from build123d import *

# Parameters (mm, degrees)
BOSS_EXTRUDE1_DEPTH     = 2.5
CUT_EXTRUDE1_DEPTH      = 37.962819157
CUT_EXTRUDE1_DEPTH_BACK = 37.962819157
SKETCH2_R               = 1


with BuildPart() as part:
    # Sketch1 → Boss-Extrude1 (new, symmetric)
    with BuildSketch(Plane(origin=(0, 0, 0), x_dir=(1, 0, 0), z_dir=(0, 1, 0))):
        Polygon((13, -6), (13, -8), (18, -8), (18, 8), (-18, 8), (-18, -8), (-13, -8), (-13, -6), (-16, -6), (-16, 6), (16, 6), (16, -6), align=None)
    extrude(amount=BOSS_EXTRUDE1_DEPTH, both=True)

    # Sketch2 → Cut-Extrude1 (cut, two sides: drawn at the far end of the back side and taken through both)
    with BuildSketch(Plane(origin=(18, 0, 0), x_dir=(0, 0, -1), z_dir=(1, 0, 0)).offset(-CUT_EXTRUDE1_DEPTH_BACK)):
        Circle(SKETCH2_R)
    extrude(amount=CUT_EXTRUDE1_DEPTH + CUT_EXTRUDE1_DEPTH_BACK, mode=Mode.SUBTRACT)


solid = part.part
CAD build for the part. Positions are in the model's coordinates, mm. A direction names the side the tool comes from. Give positions to 0.01 mm unless a question says otherwise; leave off trailing zeros. Write each loop counter-clockwise with the first axis right and the second up, starting at its lowest first coordinate (ties: lowest second). Pieces come first, ordered by that corner, then holes. Notation, with made-up numbers: (-3.5, 31.5) -> (15.5, 31.5) arc R12 cw to (15.5, 54.5) -> close; hole circle Ø8 at (-36, 9). An arc over 180 degrees is marked (long way). Return JSON: item names as keys, results as strings.
Item 1: Two-plate mould, pull along Z, no slides. Class faces 4 (the flat face through (-18, 1.15, -0.11)), 5 (the flat face through (15, 0, 8)), 6 (the flat face through (15, 0, 6)): +Z half, -Z half, draft (parallel to the pull), parting line (faces both ways), or undercut.
Answer below:
{"face 4": "draft", "face 5": "+Z half", "face 6": "undercut"}
Item 2: Band-saw the part on C-C (y = 0). List the corners of the cut face in (x, z).
Answer below:
{"outline": "(-18, -8) -> (18, -8) -> (18, -1) -> (16, -1) -> (16, -6) -> (-16, -6) -> (-16, -1) -> (-18, -1) -> close; (-18, 1) -> (-16, 1) -> (-16, 6) -> (-13, 6) -> (-13, 8) -> (-18, 8) -> close; (13, 6) -> (16, 6) -> (16, 1) -> (18, 1) -> (18, 8) -> (13, 8) -> close"}
Item 3: Band-saw the part on D-D (x = 4.5). List the corners of the cut face in (y, z).
Answer below:
{"outline": "(-2.5, -8) -> (2.5, -8) -> (2.5, -6) -> (-2.5, -6) -> close"}
Item 4: Drill centre lines: probe 1 along X at (y, z) = (-0.25, 2); probe 2 along Z at (x, y) = (17.2, 0); probe 3 along Y at (x, z) = (16.7, 0). Where is each one in solid material? Low to high.
Answer below:
{"probe 1": "x = -18 to -16, 16 to 18", "probe 2": "z = -8 to -1, 1 to 8", "probe 3": "y = -2.5 to -1, 1 to 2.5"}
Item 5: Band-saw the part on A-A (z = 0). List the corners of the cut face in (x, y).
Answer below:
{"outline": "(-18, -2.5) -> (-16, -2.5) -> (-16, -1) -> (-18, -1) -> close; (-18, 1) -> (-16, 1) -> (-16, 2.5) -> (-18, 2.5) -> close; (16, -2.5) -> (18, -2.5) -> (18, -1) -> (16, -1) -> close; (16, 1) -> (18, 1) -> (18, 2.5) -> (16, 2.5) -> close"}
Item 6: Band-saw the part on B-B (x = 14). List the corners of the cut face in (y, z), then the cut area to 3 significant figures.
Answer below:
{"outline": "(-2.5, -8) -> (2.5, -8) -> (2.5, -6) -> (-2.5, -6) -> close; (-2.5, 6) -> (2.5, 6) -> (2.5, 8) -> (-2.5, 8) -> close", "area": "20.0 mm2"}
Item 7: Tool access for faces 1 (the flat face through (16, 1.15, -0.08)), 2 (the flat face through (-13, 0, 7)), 3 (the flat face through (-1, 2.5, -7)): list every direction of +Z, -Z, +X, -X, +Y, -Y with a clear straight run to the whole face (end or side of a thin tool).
Answer below:
{"face 1": "+Y, -Y", "face 2": "+Z, +Y, -Y", "face 3": "+Z, -Z, +X, -X, +Y"}
Item 8: Drop a flat-ended pin along its axis: pin 1 (2 mm diameter, centred on x = -11.5, y = -2, fed in from +Z). Give the stop position or say it passes through.
Answer below:
{"pin 1": "stops at z = -6"}
